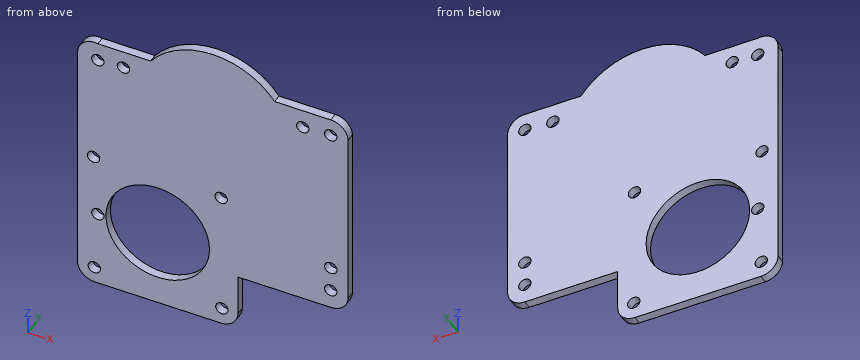
from build123d import *

# Parameters (mm, degrees)
F0_R     = 2.286
F0_R_2   = 19.1135
F1_DEPTH = 3.175


with BuildPart() as f1:
    # F0 (on Front) → F1 (new body)
    with BuildSketch(Plane.XZ):
        with BuildLine():
            Line((-15.281446, 47.29228), (-34.763334, 47.29228))
            ThreePointArc((-34.763334, 47.29228), (-39.972318, 45.923525), (-42.256334, 41.045997))
            Line((-42.256334, 41.045997), (-42.256334, -48.587158))
            ThreePointArc((-42.256334, -48.587158), (-40.396462, -53.077286), (-35.906334, -54.937158))
            Line((-35.906334, -54.937158), (10.575666, -54.937158))
            ThreePointArc((10.575666, -54.937158), (15.065794, -53.077286), (16.925666, -48.587158))
            Line((16.925666, -48.587158), (16.925666, -32.87012))
            Line((16.925666, -32.87012), (51.241066, -32.87012))
            ThreePointArc((51.241066, -32.87012), (55.731194, -31.010248), (57.591066, -26.52012))
            Line((57.591066, -26.52012), (57.591066, 40.94228))
            ThreePointArc((57.591066, 40.94228), (55.731194, 45.432408), (51.241066, 47.29228))
            Line((51.241066, 47.29228), (30.514578, 47.29228))
            ThreePointArc((30.514578, 47.29228), (7.616566, 58.77308), (-15.281446, 47.29228))
        make_face()
        with Locations((-36.083831, -48.764958)):
            Circle(F0_R, mode=Mode.SUBTRACT)
        with Locations((-34.763334, -25.58032)):
            Circle(F0_R, mode=Mode.SUBTRACT)
        with Locations((-36.354786, -1.657008)):
            Circle(F0_R, mode=Mode.SUBTRACT)
        with Locations((-12.665334, -25.075505)):
            Circle(F0_R_2, mode=Mode.SUBTRACT)
        with Locations((11.024119, -48.494002)):
            Circle(F0_R, mode=Mode.SUBTRACT)
        with Locations((10.753163, -1.386053)):
            Circle(F0_R, mode=Mode.SUBTRACT)
        with Locations((51.215666, -25.58032)):
            Circle(F0_R, mode=Mode.SUBTRACT)
        with Locations((51.215666, -16.045962)):
            Circle(F0_R, mode=Mode.SUBTRACT)
        with Locations((-34.763334, 40.25648)):
            Circle(F0_R, mode=Mode.SUBTRACT)
        with Locations((-25.331567, 40.678487)):
            Circle(F0_R, mode=Mode.SUBTRACT)
        with Locations((40.877866, 40.25648)):
            Circle(F0_R, mode=Mode.SUBTRACT)
        with Locations((51.215666, 40.678487)):
            Circle(F0_R, mode=Mode.SUBTRACT)
    extrude(amount=F1_DEPTH)


solid = f1.part
Geometry: final body of the model. Coordinates: model frame, mm. Give positions to 0.01 mm unless a question says otherwise; leave off trailing zeros. Write each loop counter-clockwise with the first axis right and the second up, starting at its lowest first coordinate (ties: lowest second). Pieces come first, ordered by that corner, then holes. Notation, with made-up numbers: (75, -29) - (98, -29) arc R14 cw to (98, -12) - close; hole circle Ø8 at (-21, 11). An arc over 180 degrees is marked (long way). Return JSON: item names as keys, results as strings. Group by question number.
1) First-contact query: P1, Ø1, axis at y = -1, z = -43, coming from the +X side; P2, Ø1.6, axis at x = 42.5, y = -2, coming from the +Z side; P3, Ø1, axis at x = 28.5, y = -1.5, coming from the -Z side; P4, Ø5.5, axis at x = 51.22, z = -25.58, coming from the -Y side (3 decimals). Flat tips, straight axial feed; report the tip coordinate or a pass-through.
2) Section B-B on y = -1.1. State how many separate pieces and enclosed holes the cut face has, plus the area to 3 significant figures.
3) Section A-A on x = -10. Return the cut outline in (y, z) (3 decimals), plus the area to 3 significant figures.
4) Section D-D on z = 51. Return the cut outline in (x, y) (3 decimals).
5) Section C-C on x = -30. Return the cut outline in (y, z) (3 decimals).
6) Line query: line 1 (X direction, y = -1.9, z = -16); line 2 (Z direction, x = 10.5, y = -0.55); line 3 (X direction, y = -2.75, z = -24). Output: solid intervals per line, ascending.
Filled in:
{
 "1": {"P1": "stops at x = 16.93", "P2": "stops at z = 47.29", "P3": "stops at z = -32.87", "P4": "stops at y = -3.175"},
 "2": {"separate pieces": "1", "enclosed holes": "12", "area": "8,310 mm^2"},
 "3": {"outline": "(-3.175, -54.937) - (0, -54.937) - (0, -44.002) - (-3.175, -44.002) - close; (-3.175, -6.149) - (0, -6.149) - (0, 52.697) - (-3.175, 52.697) - close", "area": "222 mm^2"},
 "4": {"outline": "(-11.975, -3.175) - (27.208, -3.175) - (27.208, 0) - (-11.975, 0) - close"},
 "5": {"outline": "(-3.175, -54.937) - (0, -54.937) - (0, -33.128) - (-3.175, -33.128) - close; (-3.175, -17.023) - (0, -17.023) - (0, 47.292) - (-3.175, 47.292) - close"},
 "6": {"line 1": "x = -42.26 to -29.49, 4.16 to 48.93, 53.5 to 57.59", "line 2": "z = -54.94 to -50.72, -46.27 to -3.66, 0.89 to 58.63", "line 3": "x = -42.26 to -36.42, -33.11 to -31.75, 6.42 to 49.56, 52.87 to 57.59"}
}
